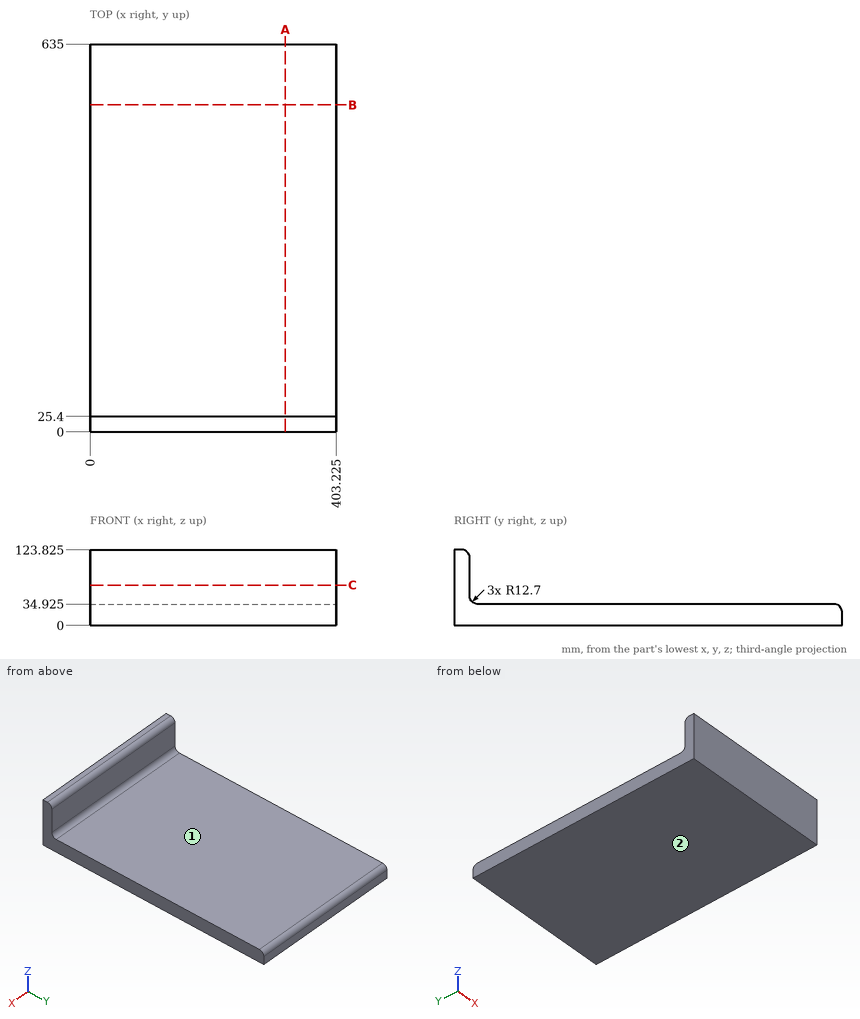
The figure shows three views and two pictorial views of one solid part (mm, origin at its lowest corner). Answer the questions. A direction names the side the tool comes from. Give positions to 0.01 mm unless a question says otherwise; leave off trailing zeros. Write each loop counter-clockwise with the first axis right and the second up, starting at its lowest first coordinate (ties: lowest second). Pieces come first, ordered by that corner, then holes. Notation, with made-up numbers: (-38, 7.25) - (-25, 7.25) arc R11 cw to (-25, 23.25) - close; hole circle Ø1 at (45, -2). An arc over 180 degrees is marked (long way). Use one line per item in the form item = value. Start each with the question number.
1) Flat-ended cylindrical pins translate along their axes: pin 1 Ø10 at (x, z) = (163.5, 42) entering from +Y; pin 2 Ø2 at (x, z) = (324, 43) entering from +Y; pin 3 Ø5 at (x, z) = (169, 71.5) entering from +Y. Find the tip coordinate at first contact, or state that the pin passes through.
2) A tool of negligible diameter and unlimited length cuts with its end or side. For the marked faces 1 and 2, from which of +Z, -Z, +X, -X, +Y, -Y can it reach the whole face along a straight path? Write none if from no direction.
3) Find section B-B on y = 535.5. Determine the outline of the cut face in (x, z) (3 decimals), plus the area to 3 significant figures.
4) Find section A-A on x = 320. Determine the outline of the cut face in (y, z) (3 decimals).
5) Find section C-C on z = 66. Determine the outline of the cut face in (x, y) (3 decimals).
6) Consider line 1 along Y through (x, z) = (109, 83); line 2 along Z through (x, y) = (297.5, 484.5) (3 decimals); line 3 along Y through (x, z) = (318, 24). Determine where each line is inside the solid, lowest interval first. Write a range as from..to.
Geometry results:
q1.pin_1 = 31.14
q1.pin_2 = 26.71
q1.pin_3 = 25.4
q2.face_1 = +Z, +X, -X, +Y
q2.face_2 = -Z, +X, -X, +Y, -Y
q3.outline = (0, 0) - (403.225, 0) - (403.225, 34.925) - (0, 34.925) - close
q3.area = 14,100 mm2
q4.outline = (0, 0) - (635, 0) - (635, 22.225) arc R12.7 ccw to (622.3, 34.925) - (38.1, 34.925) arc R12.7 cw to (25.4, 47.625) - (25.4, 111.125) arc R12.7 ccw to (12.7, 123.825) - (0, 123.825) - close
q5.outline = (0, 0) - (403.225, 0) - (403.225, 25.4) - (0, 25.4) - close
q6.line_1 = 0..25.4
q6.line_2 = 0..34.925
q6.line_3 = 0..634.88
